Read the model definition and answer for the solid it produces. Units are mm, in the model's axes. Face numbers are marked on the shaded views. A direction names the side the tool comes from. Coordinates: 2 decimals unless noted, no trailing zeros. Loops run counter-clockwise (first coordinate to the right, second up) from the corner with the lowest first, then second, coordinate; pieces in that order, holes last. Notation, with made-up numbers: M -0.75,-28.75 L 7.25,-28.75 A35 ccw 7.25,4.25 Z; hole C -21.75,-13 d3. An arc over 180 degrees is marked long. One line per item, written item: value. Start each with the question number.
```python
from build123d import *

# Parameters (mm, degrees)
MODEL_R             = 1.7499965
MODEL_R_2           = 7.75
BOSS_EXTRUDE1_DEPTH = 8
FILLET1_R           = 3
SKETCH1_W           = 14
SKETCH1_H           = 4.8
SKETCH1_R           = 0.875
BOSS_EXTRUDE2_DEPTH = 8
FILLET2_R           = 2


with BuildPart() as part:
    # Model → Boss-Extrude1 (new body)
    with BuildSketch(Plane.XY):
        Polygon((20.40532142, 11.78), (-20.40532142, 11.78), (0, -23.563053444), align=None)
        with Locations((0, -16.5)):
            Circle(MODEL_R, mode=Mode.SUBTRACT)
        Circle(MODEL_R_2, mode=Mode.SUBTRACT)
        with Locations((-14.289419163, 8.25)):
            Circle(MODEL_R, mode=Mode.SUBTRACT)
        with Locations((14.289419163, 8.25)):
            Circle(MODEL_R, mode=Mode.SUBTRACT)
    extrude(amount=BOSS_EXTRUDE1_DEPTH)

    # Fillet1
    fillet1_edges = [part.edges().sort_by_distance(p)[0] for p in [
        (0, -23.563053444, 4),
        (-20.40532142, 11.78, 4),
        (20.40532142, 11.78, 4),
    ]]
    fillet(fillet1_edges, radius=FILLET1_R)

    # Sketch1 → Boss-Extrude2 (add)
    with BuildSketch(Plane(origin=(0, 0, 0), x_dir=(-1, 0, 0), z_dir=(0, 0, -1))):
        with Locations((0, 14.18)):
            Rectangle(SKETCH1_W, SKETCH1_H)
        with Locations((-1.5, 14.18)):
            Circle(SKETCH1_R, mode=Mode.SUBTRACT)
        with Locations((-4.5, 14.18)):
            Circle(SKETCH1_R, mode=Mode.SUBTRACT)
        with Locations((1.5, 14.18)):
            Circle(SKETCH1_R, mode=Mode.SUBTRACT)
        with Locations((4.5, 14.18)):
            Circle(SKETCH1_R, mode=Mode.SUBTRACT)
    extrude(amount=-BOSS_EXTRUDE2_DEPTH)

    # Fillet2
    fillet2_edges = [part.edges().sort_by_distance(p)[0] for p in [
        (-7, 11.78, 4),
        (7, 11.78, 4),
        (7, 16.58, 4),
        (-7, 16.58, 4),
    ]]
    fillet(fillet2_edges, radius=FILLET2_R)


solid = part.part
```
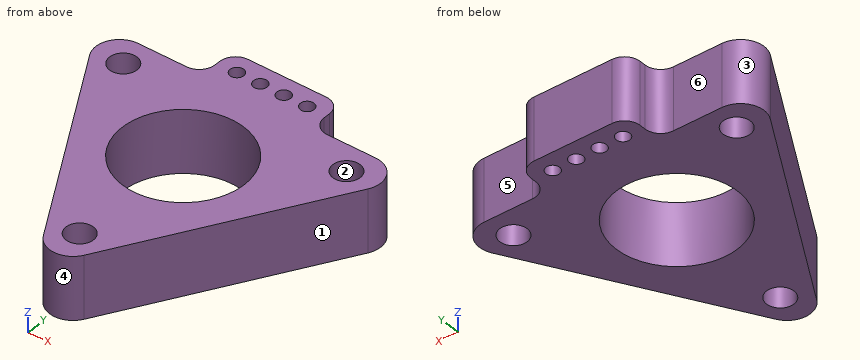
1) Consider line 1 along Y through (x, z) = (1.5, 1.5) (3 decimals); line 2 along X through (y, z) = (7, 4); line 3 along X through (y, z) = (8.5, 1). Determine where each line is inside the solid, lowest interval first.
2) Section A-A (z = 5.25) is taken. Count the separate pieces of the cut face and the enclosed holes in it, then the cut area to 3 significant figures.
3) A tool of negligible diameter and unlimited length cuts with its end or side. For the marked faces 4, 5 and 6, from which of +Z, -Z, +X, -X, +Y, -Y can it reach the whole face along a straight path? Write none if from no direction.
4) Flat-ended cylindrical pins translate along their axes: pin 1 (3 mm diameter, centred on x = 13, z = 4.5, fed in from +Y); pin 2 (1.6 mm diameter, centred on x = 4.5, y = 14.18, fed in from -Z); pin 3 (0.9 mm diameter, centred on y = 14.5, z = 2.5, fed in from -X); pin 4 (1 mm diameter, centred on x = 12, z = 1, fed in from -Y). Find the tip coordinate at first contact, or state that the pin passes through.
5) Section D-D (y = 8.25) is taken. Determine the outline of the cut face in (x, z).
6) For a pull along X with two mould halves and no side action, classify the marked faces 1, 2 and 3 as released by +X, released by -X, zero draft, split by the parting line, or undercut.
7) Section C-C (x = -4.5) is taken. Determine the outline of the cut face in (y, z) (3 decimals), then the cut area to 3 significant figures.
8) Section B-B (y = -16.5) is taken. Determine the outline of the cut face in (x, z), then the cut area to 3 significant figures.
Results found:
1. line 1: y = -20.161 to -17.401, -15.599 to -7.603, 7.603 to 13.305, 15.055 to 16.58
1. line 2: x = -17.65 to -15.51, -13.06 to -3.33, 3.33 to 13.06, 15.51 to 17.65
1. line 3: x = -18.2 to -16.02, -12.56 to 12.56, 16.02 to 18.2
2. separate pieces: 1
2. enclosed holes: 8
2. area: 543 mm²
3. face 4: +Z, -Z, -Y
3. face 5: +Z, -Z, +X, +Y
3. face 6: +Z, -Z, -X, +Y
4. pin 1: stops at y = 11.78
4. pin 2: passes through
4. pin 3: stops at x = -7
4. pin 4: stops at y = -3.64
5. outline: M -18.16,0 L -16.04,0 L -16.04,8 L -18.16,8 Z; M -12.54,0 L 12.54,0 L 12.54,8 L -12.54,8 Z; M 16.04,0 L 18.16,0 L 18.16,8 L 16.04,8 Z
6. face 1: released by +X
6. face 2: undercut
6. face 3: released by -X
7. outline: M -15.769,0 L -6.31,0 L -6.31,8 L -15.769,8 Z; M 6.31,0 L 13.305,0 L 13.305,8 L 6.31,8 Z; M 15.055,0 L 16.58,0 L 16.58,8 L 15.055,8 Z
7. area: 144 mm²
8. outline: M -4.08,0 L -1.75,0 L -1.75,8 L -4.08,8 Z; M 1.75,0 L 4.08,0 L 4.08,8 L 1.75,8 Z
8. area: 37.2 mm²
